from build123d import *

# Parameters (mm, degrees)
F0_R     = 11.1125
F1_DEPTH = 44.45
F2_R     = 6.35
F3_DEPTH = 88.9
F4_R     = 2.413
F5_DEPTH = 25.4
F6_R     = 2.413
F7_DEPTH = 25.4


with BuildPart() as f1:
    # F0 (on Front) → F1 (new body, symmetric)
    with BuildSketch(Plane.XZ):
        Circle(F0_R)
    extrude(amount=F1_DEPTH, both=True)

    # F2 (on face) → F3 (cut)
    with BuildSketch(Plane.XZ.offset(44.45)):
        Circle(F2_R)
    extrude(amount=-F3_DEPTH, mode=Mode.SUBTRACT)

    # F4 (on Right) → F5 (cut)
    with BuildSketch(Plane.YZ):
        with Locations((-29.337, 0)):
            Circle(F4_R)
    extrude(amount=-F5_DEPTH, mode=Mode.SUBTRACT)

    # F6 (on Right) → F7 (cut)
    with BuildSketch(Plane.YZ):
        with Locations((34.163, 0)):
            Circle(F6_R)
    extrude(amount=-F7_DEPTH, mode=Mode.SUBTRACT)


solid = f1.part
Geometry check sheet. Reference: the model listing, model coordinates, mm. A direction names the side the tool comes from. Give positions to 0.01 mm unless a question says otherwise; leave off trailing zeros. Order: outer loops, then holes, each group sorted by start corner. A loop starts at its lowest first (then second) coordinate and runs counter-clockwise, first axis right, second up. Notation, with made-up numbers: M 60,57 L 117,57 A26 cw 117,89 Z; hole C 57,24 d1. An arc over 180 degrees is marked long. Use a Markdown table: item, result.
Item 1: Material ranges on line 1 along X through (y, z) = (13, 0); line 2 along Z through (x, y) = (2, -27.5), recorded low to high.
Answers follow:
| item | result |
|---|---|
| line 1 | x = -11.11 to -6.35, 6.35 to 11.11 |
| line 2 | z = -10.93 to -6.03, 6.03 to 10.93 |
Item 2: Section check B-B (z = 0). Record the cut outline in (x, y).
Answers follow:
| item | result |
|---|---|
| outline | M -11.11,-44.45 L -6.35,-44.45 L -6.35,-31.75 L -11.11,-31.75 Z; M -11.11,-26.92 L -6.35,-26.92 L -6.35,31.75 L -11.11,31.75 Z; M -11.11,36.58 L -6.35,36.58 L -6.35,44.45 L -11.11,44.45 Z; M 6.35,-44.45 L 11.11,-44.45 L 11.11,44.45 L 6.35,44.45 Z |
Item 3: Section check C-C (z = -3.75). Record the cut outline in (x, y), and give its area (3 significant figures).
Answers follow:
| item | result |
|---|---|
| outline | M -10.46,-44.45 L -5.12,-44.45 L -5.12,44.45 L -10.46,44.45 Z; M 5.12,-44.45 L 10.46,-44.45 L 10.46,44.45 L 5.12,44.45 Z |
| area | 949 mm2 |
Item 4: Section check A-A (x = 0). Record the cut outline in (y, z), and give its area (3 significant figures).
Answers follow:
| item | result |
|---|---|
| outline | M -44.45,-11.11 L 44.45,-11.11 L 44.45,-6.35 L -44.45,-6.35 Z; M -44.45,6.35 L 44.45,6.35 L 44.45,11.11 L -44.45,11.11 Z |
| area | 847 mm2 |
Item 5: Depth check by flat-ended pin: P1, Ø2, axis at x = -3, z = -2.5, coming from the -Y side; P2, Ø8, axis at y = -8, z = -0.5, coming from the +X side; P3, Ø5, axis at y = -34.5, z = 8, coming from the +X side; P4, Ø3, axis at x = -6, y = 24, coming from the -Z side. Enter the tip coordinate at first touch or a pass-through.
Answers follow:
| item | result |
|---|---|
| P1 | passes through |
| P2 | stops at x = 11.11 |
| P3 | stops at x = 9.66 |
| P4 | stops at z = -10.16 |
Item 6: Draft check along Z on faces 1 (the cylindrical face through (10.265, -0.622, -4.256)), 2 (the flat face through (5, -44.45, -5)), 3 (the cylindrical face through (6.057, -0.622, 1.907)). Enter one of: +Z half, -Z half, draft (parallel to the pull), parting line (faces both ways), or undercut.
Answers follow:
| item | result |
|---|---|
| face 1 | parting line |
| face 2 | draft |
| face 3 | undercut |
Item 7: Tool access check on faces 4 (the flat face through (5, 44.45, -5)), 5 (the cylindrical face through (-8.456, -27.035, 0.725)). Record the directions out of +Z, -Z, +X, -X, +Y, -Y that give a thin tool (end or side, any length) a straight path to the whole face; none if there is none.
Answers follow:
| item | result |
|---|---|
| face 4 | +Z, -Z, +X, -X, +Y |
| face 5 | -X |
